Source: CAD feature listing. Evaluate the final solid. Frame: model axes, mm. Face numbers are marked on the shaded views. A direction names the side the tool comes from. Give positions to 0.01 mm unless a question says otherwise; leave off trailing zeros. Order: outer loops, then holes, each group sorted by start corner. A loop starts at its lowest first (then second) coordinate and runs counter-clockwise, first axis right, second up. Notation, with made-up numbers: (54, -15) -> (89, -15) arc R13 ccw to (89, 8) -> close; hole circle Ø1 at (-28, 36.25). An arc over 180 degrees is marked (long way). Use one line per item in the form item = value. Start each with the question number.
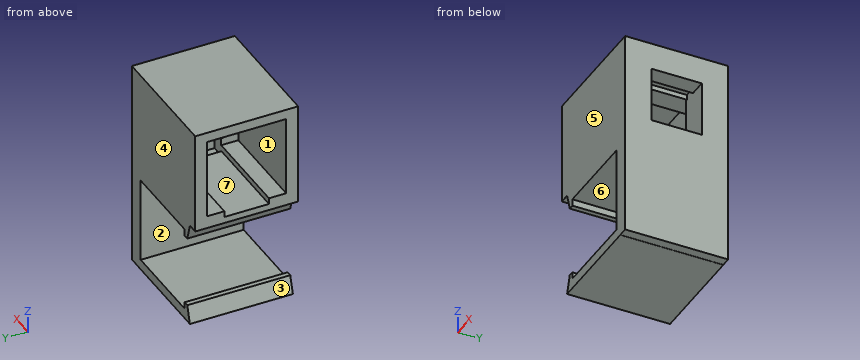
from build123d import *

# Parameters (mm, degrees)
EXTRUDE_1_DEPTH      = 30
CUT_EXTRUDE_4_DEPTH  = 82.16997337
SKETCH_7_W           = 16.60831278
SKETCH_7_H           = 38.473598513
CUT_EXTRUDE_14_DEPTH = 82.16997337
SKETCH_8_W           = 5
SKETCH_8_H           = 30.968526609
EXTRUDE_2_DEPTH      = 30
SKETCH_9_W           = 33.026813651
SKETCH_9_H           = 30
EXTRUDE_3_DEPTH      = 30
SKETCH_10_W          = 16.2
SKETCH_10_H          = 14.625
CUT_EXTRUDE_15_DEPTH = 57.68909173
SKETCH_11_W          = 23.4
SKETCH_11_H          = 23
CUT_EXTRUDE_16_DEPTH = 24.17681365
SKETCH_13_W          = 3.4
SKETCH_13_H          = 14.625
CUT_EXTRUDE_17_DEPTH = 1.5
EXTRUDE_4_DEPTH      = 5.5
SKETCH_15_W          = 4
SKETCH_15_H          = 13
CUT_EXTRUDE_18_DEPTH = 28.02681365
SKETCH_16_W          = 4
SKETCH_16_H          = 13
CUT_EXTRUDE_19_DEPTH = 1.5
SKETCH_17_W          = 30
SKETCH_17_H          = 30
EXTRUDE_5_DEPTH      = 3


with BuildPart() as part:
    # Эскиз1 → Бобышка-Вытянуть1 (new body)
    with BuildSketch(Plane(origin=(0, 0, 0), x_dir=(1, 0, 0), z_dir=(0, 1, 0))):
        Polygon((-66.825757576, 34.969739794), (-66.825757576, 29.969739794), (-63.825757576, 29.969739794), (-63.825757576, 31.969739794), (-38.825757576, 31.969739794), (-38.825757576, 6.969739794), (-63.825757576, 6.969739794), (-63.825757576, 8.969739794), (-66.825757576, 8.969739794), (-66.825757576, 3.969739794), (-22.123470102, 3.969739794), (-36.579007505, 34.969739794), align=None)
    extrude(amount=EXTRUDE_1_DEPTH)

    # Эскиз3 → Вырез-Вытянуть4 (cut, through all)
    with BuildSketch(Plane.XZ):
        Polygon((-66.825757576, -3.969739794), (-65.325757576, -8.969739794), (-66.825757576, -8.969739794), align=None)
        Polygon((-66.825757576, -29.969739794), (-66.825757576, -34.969739794), (-65.325757576, -29.969739794), align=None)
    extrude(amount=-CUT_EXTRUDE_4_DEPTH, mode=Mode.SUBTRACT)

    # Эскиз7 → Вырез-Вытянуть14 (cut, through all)
    with BuildSketch(Plane(origin=(0, 0, 0), x_dir=(-1, 0, 0), z_dir=(0, -1, 0))):
        with Locations((27.703474463, 20.539743139)):
            Rectangle(SKETCH_7_W, SKETCH_7_H)
    extrude(amount=-CUT_EXTRUDE_14_DEPTH, mode=Mode.SUBTRACT)

    # Эскиз8 → Бобышка-Вытянуть2 (add)
    with BuildSketch(Plane(origin=(0, 0, 0), x_dir=(-1, 0, 0), z_dir=(0, -1, 0))):
        with Locations((36.298943925, 19.454003098)):
            Rectangle(SKETCH_8_W, SKETCH_8_H)
    extrude(amount=-EXTRUDE_2_DEPTH)

    # Эскиз9 → Бобышка-Вытянуть3 (add)
    with BuildSketch(Plane.XY.offset(-3.969739794)):
        with Locations((-50.312350751, 15)):
            Rectangle(SKETCH_9_W, SKETCH_9_H)
    extrude(amount=EXTRUDE_3_DEPTH)

    # Эскиз10 → Вырез-Вытянуть15 (cut, through all)
    with BuildSketch(Plane(origin=(-33.798943925, 0, 0), x_dir=(0, 0, -1), z_dir=(1, 0, 0))):
        with Locations((-10.030260206, 14.9975)):
            Rectangle(SKETCH_10_W, SKETCH_10_H)
    extrude(amount=-CUT_EXTRUDE_15_DEPTH, mode=Mode.SUBTRACT)

    # Эскиз11 → Вырез-Вытянуть16 (cut)
    with BuildSketch(Plane.ZY.offset(66.825757576)):
        with Locations((11.430260206, 15)):
            Rectangle(SKETCH_11_W, SKETCH_11_H)
    extrude(amount=-CUT_EXTRUDE_16_DEPTH, mode=Mode.SUBTRACT)

    # Эскиз13 → Вырез-Вытянуть17 (cut)
    with BuildSketch(Plane(origin=(0, 0, 18.130260206), x_dir=(-1, 0, 0), z_dir=(0, 0, -1))):
        with Locations((40.498943925, 14.9975)):
            Rectangle(SKETCH_13_W, SKETCH_13_H)
    extrude(amount=-CUT_EXTRUDE_17_DEPTH, mode=Mode.SUBTRACT)

    # Эскиз14 → Бобышка-Вытянуть4 (add)
    with BuildSketch(Plane.ZY.offset(42.648943925)):
        Polygon((18.130260206, 22.31), (18.130260206, 26.5), (23.130260206, 26.5), (23.130260206, 3.5), (18.130260206, 3.5), (18.130260206, 7.685), align=None)
    extrude(amount=EXTRUDE_4_DEPTH)

    # Эскиз15 → Вырез-Вытянуть18 (cut)
    with BuildSketch(Plane.ZY.offset(66.825757576)):
        with Locations((-0.069739794, 15)):
            Rectangle(SKETCH_15_W, SKETCH_15_H)
    extrude(amount=-CUT_EXTRUDE_18_DEPTH, mode=Mode.SUBTRACT)

    # Эскиз16 → Вырез-Вытянуть19 (cut)
    with BuildSketch(Plane.XY.offset(-2.069739794)):
        with Locations((-40.798943925, 15)):
            Rectangle(SKETCH_16_W, SKETCH_16_H)
    extrude(amount=-CUT_EXTRUDE_19_DEPTH, mode=Mode.SUBTRACT)

    # Эскиз17 → Бобышка-Вытянуть5 (add)
    with BuildSketch(Plane.ZY.offset(66.825757576)):
        with Locations((11.030260206, 15)):
            Rectangle(SKETCH_17_W, SKETCH_17_H)
        Polygon((-0.269739794, 26.5), (23.130260206, 26.5), (23.130260206, 3.5), (-0.269739794, 3.5), (-0.269739794, 8.5), (-2.069739794, 8.5), (-2.069739794, 21.5), (-0.269739794, 21.5), align=None, mode=Mode.SUBTRACT)
    extrude(amount=EXTRUDE_5_DEPTH)


solid = part.part
1) Reachability of the marked faces 1, 2 and 3 from +Z, -Z, +X, -X, +Y, -Y: full face, straight path, thin tool, end or side. Return the list, or none.
2) Cut plane A-A, the plane x = -40. Return the cut outline in (y, z) (3 decimals).
3) Draft query along Y for the marked faces 4, 5, 6 and 7. Return one class per face: +Y half, -Y half, draft (parallel to the pull), parting line (faces both ways), or undercut.
4) Material intervals for probe 1 along Z at (x, y) = (-56.5, 14); probe 2 along Z at (x, y) = (-39, 8); probe 3 along Y at (x, z) = (-48.5, 14.5), sorted ascending.
5) Cut plane B-B, the plane z = 15.5. Return the cut outline in (x, y) (3 decimals), plus the area to 3 significant figures.
Output values:
q1.face_1 = -X
q1.face_2 = +Y, -Y
q1.face_3 = -X, +Y, -Y
q2.outline = (0, -34.97) -> (30, -34.97) -> (30, -31.97) -> (0, -31.97) -> close; (0, -6.97) -> (30, -6.97) -> (30, 26.03) -> (0, 26.03) -> close; hole (7.685, 1.93) -> (8.5, 1.93) -> (8.5, -3.57) -> (21.5, -3.57) -> (21.5, 1.93) -> (22.31, 1.93) -> (22.31, 19.63) -> (7.685, 19.63) -> close
q3.face_4 = +Y half
q3.face_5 = -Y half
q3.face_6 = draft
q3.face_7 = undercut
q4.probe_1 = -34.97 to -31.97, -6.97 to -2.07, 23.13 to 26.03
q4.probe_2 = -34.97 to -31.97, -6.97 to 1.93, 19.63 to 26.03
q4.probe_3 = 0 to 3.5, 26.5 to 30
q5.outline = (-69.826, 0) -> (-33.799, 0) -> (-33.799, 7.685) -> (-42.649, 7.685) -> (-42.649, 3.5) -> (-69.826, 3.5) -> close; (-69.826, 26.5) -> (-42.649, 26.5) -> (-42.649, 22.31) -> (-33.799, 22.31) -> (-33.799, 30) -> (-69.826, 30) -> close
q5.area = 326 mm^2
